from build123d import *

# Parameters (mm, degrees)
SKETCH1_W                                     = 254
SKETCH1_H                                     = 25.4
BOSS_EXTRUDE1_DEPTH                           = 6.35
CSK_FOR_1_4_FLAT_HEAD_MACHINE_SCREW1_AT_COUNT = 2
CSK_FOR_1_4_FLAT_HEAD_MACHINE_SCREW1_AT_PITCH = 228.6
CSK_FOR_1_4_FLAT_HEAD_MACHINE_SCREW1_2_COUNT  = 2
CSK_FOR_1_4_FLAT_HEAD_MACHINE_SCREW1_2_PITCH  = 114.3


with BuildPart() as part:
    # Sketch1 → Boss-Extrude1 (new body)
    with BuildSketch(Plane(origin=(0, 0, 0), x_dir=(1, 0, 0), z_dir=(0, 1, 0))):
        with Locations((-127, 12.7)):
            Rectangle(SKETCH1_W, SKETCH1_H)
    extrude(amount=BOSS_EXTRUDE1_DEPTH)

    # Sketch7 → CSK for 1/4 Flat Head Machine Screw1 (revolve, cut)
    with BuildSketch(Plane(origin=(-241.3, 0, -12.7), x_dir=(0, 0, -1), z_dir=(1, 0, 0))):
        Polygon((0, 0), (0, 6.35), (3.2639, 6.35), (3.2639, 3.652419693), (6.4389, 0), align=None)
    csk_for_1_4_flat_head_machine_screw1 = revolve(axis=Axis((-241.3, -6.35, -12.7), (0, 1, 0)), mode=Mode.SUBTRACT)

    # CSK for 1/4 Flat Head Machine Screw1 at: CSK for 1/4 Flat Head Machine Screw1 ×2
    with Locations(*[(i * CSK_FOR_1_4_FLAT_HEAD_MACHINE_SCREW1_AT_PITCH, 0, 0) for i in range(1, CSK_FOR_1_4_FLAT_HEAD_MACHINE_SCREW1_AT_COUNT)]):
        add(csk_for_1_4_flat_head_machine_screw1, mode=Mode.SUBTRACT)

    # CSK for 1_4 Flat Head Machine Screw1 2: CSK for 1/4 Flat Head Machine Screw1 ×2
    with Locations(*[(i * CSK_FOR_1_4_FLAT_HEAD_MACHINE_SCREW1_2_PITCH, 0, 0) for i in range(1, CSK_FOR_1_4_FLAT_HEAD_MACHINE_SCREW1_2_COUNT)]):
        add(csk_for_1_4_flat_head_machine_screw1, mode=Mode.SUBTRACT)


solid = part.part
Can you work these out from the model? Positions are in its coordinate system, mm. Round coordinates to 2 decimals unless told otherwise and drop trailing zeros. Write each loop counter-clockwise with the first axis right and the second up, starting at its lowest first coordinate (ties: lowest second). Pieces come first, ordered by that corner, then holes. Notation, with made-up numbers: (80, -31) -> (133, -31) arc R16 cw to (133, -10) -> close; hole circle Ø7 at (41.25, 48.5). An arc over 180 degrees is marked (long way). Use one line per item in the form item = value. Start each with the question number.
Q1. Imagine slicing it at B-B (y = 5). Please give me the cut outline in (x, z), then the cut area to 3 significant figures.
Q2. We'd pull the mould along X, two halves only. Please class faces 1 (the face through (-129, 6.35, -16)), 2 (the face through (0, 3, -13)), 3 (the face through (-254, 3, -13)), 4 (the face through (-244.536, 4.982, -12.275)): +X half, -X half, draft (parallel to the pull), parting line (faces both ways), or undercut.
Q3. Imagine slicing it at C-C (z = -12.7). Please give me the cut outline in (x, y).
Q4. Imagine slicing it at A-A (x = -241.3). Please give me the cut outline in (y, z), then the cut area to 3 significant figures.
Q5. If I drill on probe 1 along X at (y, z) = (4.8, -12.7); probe 2 along Z at (x, y) = (-127, 4.85); probe 3 along X at (y, z) = (2.5, -12.5), over which ranges is the centre line in solid material (lowest first)? Write a range as [from, to].
Q6. I'm going to push flat-ended pins straight in: P1, Ø8, axis at x = -79.5, z = -9.5, coming from the -Y side; P2, Ø4, axis at x = -241.3, z = -12.7, coming from the -Y side; P3, Ø10.5, axis at x = -12.7, z = -12.7, coming from the -Y side. Where does each tip first touch, or does it pass through?
Worked out:
q1.outline = (-254, -25.4) -> (0, -25.4) -> (0, 0) -> (-254, 0) -> close; hole circle Ø6.53 at (-241.3, -12.7); hole circle Ø6.53 at (-127, -12.7); hole circle Ø6.53 at (-12.7, -12.7)
q1.area = 6,350 mm^2
q2.face_1 = draft
q2.face_2 = +X half
q2.face_3 = -X half
q2.face_4 = undercut
q3.outline = (-254, 0) -> (-247.74, 0) -> (-244.56, 3.65) -> (-244.56, 6.35) -> (-254, 6.35) -> close; (-238.04, 3.65) -> (-234.86, 0) -> (-133.44, 0) -> (-130.26, 3.65) -> (-130.26, 6.35) -> (-238.04, 6.35) -> close; (-123.74, 3.65) -> (-120.56, 0) -> (-19.14, 0) -> (-15.96, 3.65) -> (-15.96, 6.35) -> (-123.74, 6.35) -> close; (-9.44, 3.65) -> (-6.26, 0) -> (0, 0) -> (0, 6.35) -> (-9.44, 6.35) -> close
q4.outline = (0, -25.4) -> (6.35, -25.4) -> (6.35, -15.96) -> (3.65, -15.96) -> (0, -19.14) -> close; (0, -6.26) -> (3.65, -9.44) -> (6.35, -9.44) -> (6.35, 0) -> (0, 0) -> close
q4.area = 108 mm^2
q5.probe_1 = [-254, -244.56], [-238.04, -130.26], [-123.74, -15.96], [-9.44, 0]
q5.probe_2 = [-25.4, -15.96], [-9.44, 0]
q5.probe_3 = [-254, -245.56], [-237.04, -131.26], [-122.74, -16.96], [-8.44, 0]
q6.P1 = 0
q6.P2 = through
q6.P3 = 1.37
